from build123d import *

# Parameters (mm, degrees)
SKETCH_W  = 120
SKETCH_H  = 60
SKETCH_R  = 20
PAD_DEPTH = 10


with BuildPart() as part:
    # Sketch → Pad (new body)
    with BuildSketch(Plane.XY):
        Rectangle(SKETCH_W, SKETCH_H)
        Circle(SKETCH_R, mode=Mode.SUBTRACT)
    extrude(amount=PAD_DEPTH)


solid = part.part
Part model, mm, in its own coordinate system. Give positions to 0.01 mm unless a question says otherwise; leave off trailing zeros. Write each loop counter-clockwise with the first axis right and the second up, starting at its lowest first coordinate (ties: lowest second). Pieces come first, ordered by that corner, then holes.
1) Probe L1, parallel to Y at x = 0, z = 4.25; L2, parallel to Y at x = -10, z = 7.75; L3, parallel to X at y = 17, z = 9. List the from-to ranges inside material, lowest first.
Resolved:
L1: y = -30 to -20, 20 to 30
L2: y = -30 to -17.32, 17.32 to 30
L3: x = -60 to -10.54, 10.54 to 60
2) Cut at C-C on z = 6.75. Write the cut outline in (x, y).
Resolved:
outline: (-60, -30) - (60, -30) - (60, 30) - (-60, 30) - close; hole circle Ø40 at (0, 0)
3) Cut at B-B on y = 12. Write the cut outline in (x, z).
Resolved:
outline: (-60, 0) - (-16, 0) - (-16, 10) - (-60, 10) - close; (16, 0) - (60, 0) - (60, 10) - (16, 10) - close
4) Cut at A-A on x = 0. Write the cut outline in (y, z), then the cut area to 3 significant figures.
Resolved:
outline: (-30, 0) - (-20, 0) - (-20, 10) - (-30, 10) - close; (20, 0) - (30, 0) - (30, 10) - (20, 10) - close
area: 200 mm2
5) Two-plate mould, pull along Y, no slides. Class faces 1 (the face through (-60, 0, 5)), 2 (the face through (-1, -30, 5)), 3 (the face through (-4.336, -19.524, 4.93)): released by +Y, released by -Y, zero draft, split by the parting line, or undercut.
Resolved:
face 1: zero draft
face 2: released by -Y
face 3: undercut
